Read the model definition and answer for the solid it produces. Units are mm, in the model's axes. Face numbers are marked on the shaded views. A direction names the side the tool comes from. Coordinates: 2 decimals unless noted, no trailing zeros. Write each loop counter-clockwise with the first axis right and the second up, starting at its lowest first coordinate (ties: lowest second). Pieces come first, ordered by that corner, then holes. Notation, with made-up numbers: (88.25, -17.5) -> (110.25, -17.5) arc R24 cw to (110.25, 0.5) -> close; hole circle Ø2 at (29.25, 21). An arc over 180 degrees is marked (long way). Answer as a JSON object with one key per item and string values. Group by question number.
(1) Find section D-D (z = -21). Give the vertices of the cut face in (x, y).
(2) Straight lines are drawn through the part: L1, parallel to Z at x = -0.75, y = 0; L2, parallel to Y at x = 0, z = 11.35; L3, parallel to Z at x = 0, y = 2.5. For each, find the intervals that lie inside material, in ascending order.
(3) Find section B-B (x = 0). Give the vertices of the cut face in (y, z).
(4) Find section A-A (y = 0). Give the vertices of the cut face in (x, z), then the cut area to 3 significant figures.
(5) Flat-ended cylindrical pins translate along their axes: P1, Ø2, axis at x = -1.5, z = -20, coming from the -Y side; P2, Ø1, axis at x = 1, y = -2.5, coming from the -Z side; P3, Ø3.5, axis at x = 0, y = 0, coming from the +Z side. Find the tip coordinate at first contact, or state that the pin passes through.
(6) Which of the six approach directions +Z, -Z, +X, -X, +Y, -Y give full straight-line access (tool end or side, diameter ignored) to the marked faces 1 and 2?
(7) Find section C-C (z = 6). Give the vertices of the cut face in (x, y), then the cut area to 3 significant figures.
from build123d import *

# Parameters (mm, degrees)
CUT_EXTRUDE_1_DEPTH      = 33.803886965
CUT_EXTRUDE_1_DEPTH_BACK = 33.803886965
SKETCH_3_R               = 1.1
CHAMFER_1_SIZE           = 0.5
CHAMFER_3_SIZE           = 0.2


with BuildPart() as part:
    # 스케치2 → 회전1 (revolve)
    with BuildSketch(Plane(origin=(0, 0, 0), x_dir=(1, 0, 0), z_dir=(0, 1, 0)), mode=Mode.PRIVATE) as revolve_1_sk:
        Polygon((0, 32.5), (0, -11), (2, -11), (2, -12), (3.15, -12), (3.15, -2), (3, -2), (3, 0), (2.1, 0), (2.1, 32.5), align=None)
    revolve(revolve_1_sk.sketch.rotate(Axis((0, 0, -32.5), (0, 0, 1)), 180), axis=Axis((0, 0, -32.5), (0, 0, 1)))

    # 스케치3 → 컷-돌출1 (cut, two sides: drawn at the far end of the back side and taken through both)
    with BuildSketch(Plane(origin=(0, 0, 0), x_dir=(0, 0, -1), z_dir=(1, 0, 0)).offset(-CUT_EXTRUDE_1_DEPTH_BACK)):
        with Locations((-6, 0)):
            Circle(SKETCH_3_R)
    extrude(amount=CUT_EXTRUDE_1_DEPTH + CUT_EXTRUDE_1_DEPTH_BACK, mode=Mode.SUBTRACT)

    # 모따기1
    chamfer_1_edges = [part.edges().sort_by_distance(p)[0] for p in [
        (2, 0, 12),
    ]]
    chamfer(chamfer_1_edges, length=CHAMFER_1_SIZE)

    # 모따기3
    # the kernel refuses this chamfer: 0.2 mm, written as the material it adds along each edge
    with BuildSketch(Plane(origin=(0, 0, 2), x_dir=(-1, 0, 0), z_dir=(0, 1, 0))) as chamfer_3_piece_1_section:
        Polygon((3 + CHAMFER_3_SIZE, 0), (3, -CHAMFER_3_SIZE), (3, 0), align=None)
    chamfer_3_piece_1 = revolve(axis=Axis((0, 0, 2), (0, 0, 1)), mode=Mode.PRIVATE)
    chamfer_3_piece_1 = chamfer_3_piece_1 & Plane(origin=(0, 0, 1.877341944), x_dir=(-1, 0, 0), z_dir=(0, 0, -1)) * Cylinder(3.15, 13, mode=Mode.PRIVATE)
    add(chamfer_3_piece_1)
    # the kernel refuses this chamfer: 0.2 mm, written as the material it takes off along each edge
    with BuildSketch(Plane(origin=(0, 0, 12), x_dir=(-1, 0, 0), z_dir=(0, 1, 0))) as chamfer_3_2_piece_1:
        Polygon((3.15 - CHAMFER_3_SIZE, 0), (3.15, -CHAMFER_3_SIZE), (3.15, 0), align=None)
    revolve(axis=Axis((0, 0, 12), (0, 0, 1)), mode=Mode.SUBTRACT)


solid = part.part
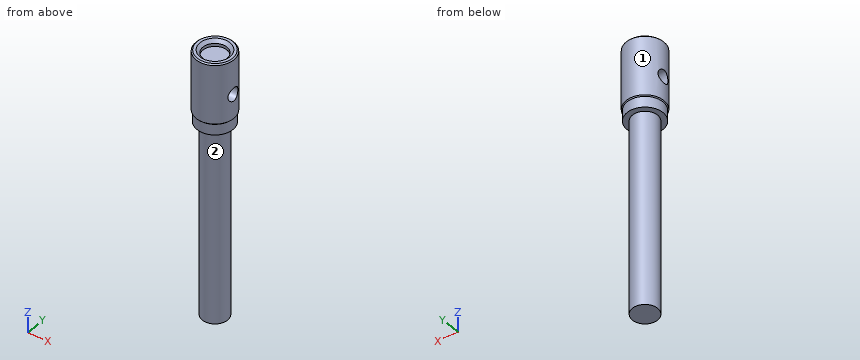
Results below:
{
 "1": {"outline": "circle Ø4.2 at (0, 0)"},
 "2": {"L1": "z = -32.5 to 4.9, 7.1 to 11", "L2": "y = -3.15 to -2, 2 to 3.15", "L3": "z = 0 to 12"},
 "3": {"outline": "(-3.15, 1.95) -> (-3, 1.8) -> (-3, 0) -> (-2.1, 0) -> (-2.1, -32.5) -> (2.1, -32.5) -> (2.1, 0) -> (3, 0) -> (3, 1.8) -> (3.15, 1.95) -> (3.15, 11.8) -> (2.95, 12) -> (2.5, 12) -> (2, 11.5) -> (2, 11) -> (-2, 11) -> (-2, 11.5) -> (-2.5, 12) -> (-2.95, 12) -> (-3.15, 11.8) -> close; hole circle Ø2.2 at (0, 6)"},
 "4": {"outline": "(-3.15, 1.95) -> (-3, 1.8) -> (-3, 0) -> (-2.1, 0) -> (-2.1, -32.5) -> (2.1, -32.5) -> (2.1, 0) -> (3, 0) -> (3, 1.8) -> (3.15, 1.95) -> (3.15, 4.9) -> (-3.15, 4.9) -> close; (-3.15, 7.1) -> (3.15, 7.1) -> (3.15, 11.8) -> (2.95, 12) -> (2.5, 12) -> (2, 11.5) -> (2, 11) -> (-2, 11) -> (-2, 11.5) -> (-2.5, 12) -> (-2.95, 12) -> (-3.15, 11.8) -> close", "area": "193 mm2"},
 "5": {"P1": "stops at y = -2.04", "P2": "stops at z = 0", "P3": "stops at z = 11"},
 "6": {"face 1": "+Z, -Z", "face 2": "-Z"},
 "7": {"outline": "(-2.95, -1.1) arc R3.15 ccw to (2.95, -1.1) -> close; (-2.95, 1.1) -> (2.95, 1.1) arc R3.15 ccw to start", "area": "17.6 mm2"}
}
